```python
from build123d import *

# Parameters (mm, degrees)
SKETCH005_W                = 29
SKETCH005_H                = 47
PAD001_DEPTH               = 1
SKETCH006_R                = 1
POCKET003_DEPTH            = 111.472716
SKETCH006_MIRRORED_2_R     = 1
POCKET003_MIRRORED_2_DEPTH = 111.472716
FILLET002_R                = 3


with BuildPart() as part:
    # Sketch005 → Pad001 (new body)
    with BuildSketch(Plane.XY):
        Rectangle(SKETCH005_W, SKETCH005_H)
    extrude(amount=PAD001_DEPTH)

    # Sketch006 (on Face6 of Pad001) → Pocket003 (cut, through all)
    with BuildSketch(Plane.XY.offset(1)):
        with Locations((-11.5, 21.5)):
            Circle(SKETCH006_R)
    pocket003 = extrude(amount=-POCKET003_DEPTH, mode=Mode.SUBTRACT)

    # Sketch006 Mirrored 2 → Pocket003 Mirrored 2 (cut, through all)
    with BuildSketch(Plane(origin=(0, 0, 1), x_dir=(-1, 0, 0), z_dir=(0, 0, -1))):
        with Locations((-11.5, 21.5)):
            Circle(SKETCH006_MIRRORED_2_R)
    pocket003_mirrored_2 = extrude(amount=POCKET003_MIRRORED_2_DEPTH, mode=Mode.SUBTRACT)

    # Mirrored001: Pocket003, Pocket003 Mirrored 2 across Sketch006 H_Axis
    add(pocket003.mirror(Plane(origin=(0, 0, 1), x_dir=(0, 0, 1), z_dir=(0, 1, 0))), mode=Mode.SUBTRACT)
    add(pocket003_mirrored_2.mirror(Plane(origin=(0, 0, 1), x_dir=(0, 0, 1), z_dir=(0, 1, 0))), mode=Mode.SUBTRACT)

    # Fillet002
    fillet002_edges = [part.edges().sort_by_distance(p)[0] for p in [
        (-14.5, -23.5, 0.5),
        (14.5, -23.5, 0.5),
        (-14.5, 23.5, 0.5),
        (14.5, 23.5, 0.5),
    ]]
    fillet(fillet002_edges, radius=FILLET002_R)


with BuildPart() as part_1:
    # Body001 placement: moved
    add(part.part.moved(Location((0, 0, 14))))


solid = part_1.part
```
CAD build for the part. Positions are in the model's coordinates, mm. Round coordinates to 2 decimals unless told otherwise and drop trailing zeros. Order: outer loops, then holes, each group sorted by start corner. A loop starts at its lowest first (then second) coordinate and runs counter-clockwise, first axis right, second up.
Item 1: Mould opens along Y. For faces 1 (the face through (-11.717, 20.524, 14.507)), 2 (the face through (0, 0, 14)), 3 (the face through (13.6, 22.64, 14.51)) say: pulls with the +Y half, pulls with the -Y half, needs draft (parallel to the pull), parting line crosses it, or undercut.
Item 2: Probe line 1 along Y through (x, z) = (11.5, 14.5); line 2 along X through (y, z) = (-21.5, 14.4); line 3 along X through (y, z) = (-21, 14.8). List the from-to ranges inside material, lowest first.
Item 3: Saw through at A-A on y = 21.5. Write the cut outline in (x, z).
Reported:
1. face 1: undercut
1. face 2: needs draft
1. face 3: pulls with the +Y half
2. line 1: y = -23.5 to -22.5, -20.5 to 20.5, 22.5 to 23.5
2. line 2: x = -14.33 to -12.5, -10.5 to 10.5, 12.5 to 14.33
2. line 3: x = -14.46 to -12.37, -10.63 to 10.63, 12.37 to 14.46
3. outline: (-14.33, 14) - (-12.5, 14) - (-12.5, 15) - (-14.33, 15) - close; (-10.5, 14) - (10.5, 14) - (10.5, 15) - (-10.5, 15) - close; (12.5, 14) - (14.33, 14) - (14.33, 15) - (12.5, 15) - close
